Job drawing, mm, ordinate dimensions from the low corner. One solid piece. Round coordinates to 2 decimals unless told otherwise and drop trailing zeros. Loops run counter-clockwise (first coordinate to the right, second up) from the corner with the lowest first, then second, coordinate; pieces in that order, holes last.
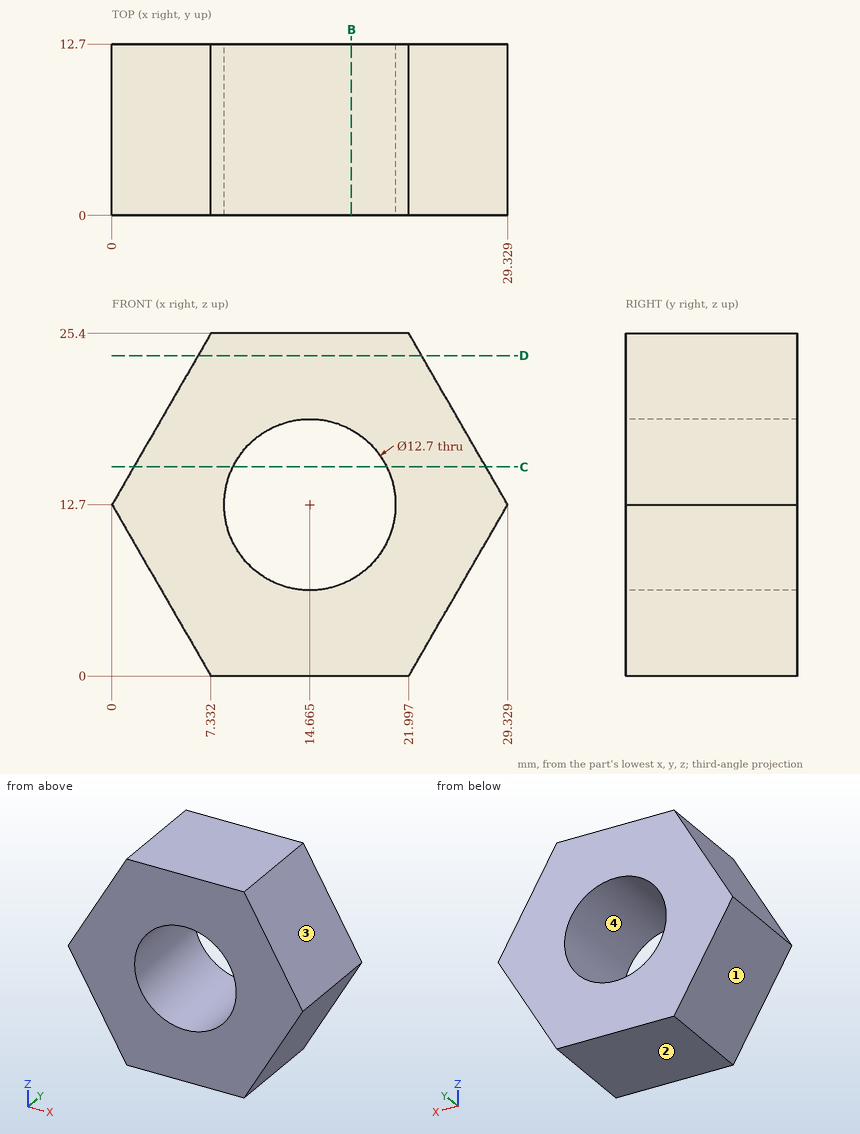
Item 1: Probe line 1 (Z direction, x = 14.5, y = 11); line 2 (Z direction, x = 18.5, y = 4.75); line 3 (Z direction, x = 3, y = 10) (1 decimal). List the from-to ranges inside material, lowest first.
Answers follow:
line 1: z = 0 to 6.35, 19.05 to 25.4
line 2: z = 0 to 7.64, 17.76 to 25.4
line 3: z = 7.5 to 17.9
Item 2: Cut at C-C, the plane z = 15.5. Give the cut face in (x, y) (1 decimal).
Answers follow:
outline: (1.6, 0) - (9, 0) - (9, 12.7) - (1.6, 12.7) - close; (20.4, 0) - (27.7, 0) - (27.7, 12.7) - (20.4, 12.7) - close
Item 3: Cut at D-D, the plane z = 23.75. Give the cut face in (x, y), plus the area to 3 significant figures.
Answers follow:
outline: (6.38, 0) - (22.95, 0) - (22.95, 12.7) - (6.38, 12.7) - close
area: 210 mm2
Item 4: Cut at B-B, the plane x = 17.75. Give the cut face in (y, z).
Answers follow:
outline: (0, 0) - (12.7, 0) - (12.7, 7.15) - (0, 7.15) - close; (0, 18.25) - (12.7, 18.25) - (12.7, 25.4) - (0, 25.4) - close
Item 5: Two-plate mould, pull along X, no slides. Class the marked faces 1, 2, 3 and 4: released by +X, released by -X, zero draft, split by the parting line, or undercut.
Answers follow:
face 1: released by -X
face 2: zero draft
face 3: released by +X
face 4: undercut
Item 6: Flat gauge pins, fed straight in: P1, Ø2, axis at y = 8, z = 18.5, coming from the -X side; P2, Ø1, axis at y = 8, z = 13.5, coming from the +X side; P3, Ø6, axis at y = 8.5, z = 8, coming from the +X side. Where does each tip first touch, or does it go through?
Answers follow:
P1: stops at x = 2.77
P2: stops at x = 29.16
P3: stops at x = 28.35
